from build123d import *

# Parameters (mm, degrees)
F0_W     = 34
F0_H     = 76
F0_W_2   = 26
F0_H_2   = 20
F1_DEPTH = 2
F2_R     = 3
F3_R     = 7
F5_DEPTH = 25


with BuildPart() as f1:
    # F0 (on Top) → F1 (new body)
    with BuildSketch(Plane.XY):
        with Locations((17, 38)):
            Rectangle(F0_W, F0_H)
        with Locations((17, 62)):
            Rectangle(F0_W_2, F0_H_2, mode=Mode.SUBTRACT)
    extrude(amount=F1_DEPTH)

    # F2
    f2_edges = [f1.edges().sort_by_distance(p)[0] for p in [
        (4, 72, 1),
        (30, 72, 1),
        (30, 52, 1),
        (4, 52, 1),
    ]]
    fillet(f2_edges, radius=F2_R)

    # F3
    f3_edges = [f1.edges().sort_by_distance(p)[0] for p in [
        (34, 76, 1),
        (0, 76, 1),
        (0, 0, 1),
        (34, 0, 1),
    ]]
    fillet(f3_edges, radius=F3_R)

    # F4 (on face) → F5 (cut)
    with BuildSketch(Plane.XY.offset(2)):
        with BuildLine():
            ThreePointArc((6.12132, 9.12132), (4.62132, 10.62132), (3.12132, 9.12132))
            ThreePointArc((3.12132, 9.12132), (4.87868, 4.87868), (9.12132, 3.12132))
            ThreePointArc((9.12132, 3.12132), (10.62132, 4.62132), (9.12132, 6.12132))
            ThreePointArc((9.12132, 6.12132), (7, 7), (6.12132, 9.12132))
        make_face()
        with BuildLine():
            Line((17.87868, 6.12132), (16.12132, 6.12132))
            ThreePointArc((16.12132, 6.12132), (14.62132, 4.62132), (16.12132, 3.12132))
            Line((16.12132, 3.12132), (17.87868, 3.12132))
            ThreePointArc((17.87868, 3.12132), (19.37868, 4.62132), (17.87868, 6.12132))
        make_face()
        with BuildLine():
            ThreePointArc((27.87868, 9.12132), (27, 7), (24.87868, 6.12132))
            ThreePointArc((24.87868, 6.12132), (23.37868, 4.62132), (24.87868, 3.12132))
            ThreePointArc((24.87868, 3.12132), (29.12132, 4.87868), (30.87868, 9.12132))
            ThreePointArc((30.87868, 9.12132), (29.37868, 10.62132), (27.87868, 9.12132))
        make_face()
    extrude(amount=-F5_DEPTH, mode=Mode.SUBTRACT)


solid = f1.part
Could you check a few things on this model? Use its own coordinates, in mm. A direction names the side the tool comes from. Coordinates: 2 decimals unless noted, no trailing zeros. Order: outer loops, then holes, each group sorted by start corner. A loop starts at its lowest first (then second) coordinate and runs counter-clockwise, first axis right, second up.
Q1. Suppose I cut it at C-C on z = 1.4. Please give me the cut outline in (x, y), and give its area (3 significant figures).
Q2. Thinking about a two-plate mould opening in Y: for faces 1 (the cylindrical face through (29.14, 71.1, 1.01)), 2 (the flat face through (17, 0, 1)), 3 (the cylindrical face through (31.9, 74, 1)), which applies, released by +Y, released by -Y, zero draft, split by the parting line, or undercut?
Q3. Suppose I cut it at D-D on y = 5. Please give me the cut outline in (x, z).
Q4. Suppose I cut it at B-B on x = 12.5. Please give me the cut outline in (y, z).
Q5. Suppose I cut it at A-A on y = 57. Please give me the cut outline in (x, z), and give its area (3 significant figures).
Q6. Please list where these lines run through material, in increasing order: L1, parallel to Y at x = 18, z = 0.4; L2, parallel to Y at x = 22, z = 1.2; L3, parallel to X at y = 66.5, z = 1.85.
Q7. Which directions (+Z, -Z, +X, -X, +Y, -Y) give clear straight access to the entire face, cutting with the end or side of a thin tool? Please do faces 4 (the flat face through (17, 39, 2)), 5 (the cylindrical face through (4.65, 10.62, 1.01)).
Answer:
1. outline: (0, 7) arc R7 ccw to (7, 0) - (27, 0) arc R7 ccw to (34, 7) - (34, 69) arc R7 ccw to (27, 76) - (7, 76) arc R7 ccw to (0, 69) - close; hole (3.12, 9.12) arc R6 ccw to (9.12, 3.12) arc R1.5 ccw to (9.12, 6.12) arc R3 cw to (6.12, 9.12) arc R1.5 ccw to start; hole (4, 55) arc R3 ccw to (7, 52) - (27, 52) arc R3 ccw to (30, 55) - (30, 69) arc R3 ccw to (27, 72) - (7, 72) arc R3 ccw to (4, 69) - close; hole (16.12, 3.12) - (17.88, 3.12) arc R1.5 ccw to (17.88, 6.12) - (16.12, 6.12) arc R1.5 ccw to start; hole (24.88, 3.12) arc R6 ccw to (30.88, 9.12) arc R1.5 ccw to (27.88, 9.12) arc R3 cw to (24.88, 6.12) arc R1.5 ccw to start
1. area: 1,960 mm2
2. face 1: undercut
2. face 2: released by -Y
2. face 3: released by +Y
3. outline: (0.29, 0) - (4.76, 0) - (4.76, 2) - (0.29, 2) - close; (10.57, 0) - (14.67, 0) - (14.67, 2) - (10.57, 2) - close; (19.33, 0) - (23.43, 0) - (23.43, 2) - (19.33, 2) - close; (29.24, 0) - (33.71, 0) - (33.71, 2) - (29.24, 2) - close
4. outline: (0, 0) - (52, 0) - (52, 2) - (0, 2) - close; (72, 0) - (76, 0) - (76, 2) - (72, 2) - close
5. outline: (0, 0) - (4, 0) - (4, 2) - (0, 2) - close; (30, 0) - (34, 0) - (34, 2) - (30, 2) - close
5. area: 16.0 mm2
6. L1: y = 0 to 3.13, 6.12 to 52, 72 to 76
6. L2: y = 0 to 52, 72 to 76
6. L3: x = 0 to 4, 30 to 34
7. face 4: +Z, +X, -X, +Y, -Y
7. face 5: +Z, -Z
